from build123d import *

# Parameters (mm, degrees)
F0_W     = 10
F0_H     = 20
F1_DEPTH = 5
F2_R     = 1.5
F2_R_2   = 2.5
F3_DEPTH = 5
F4_R     = 1


with BuildPart() as f1:
    # F0 (on Top) → F1 (new body)
    with BuildSketch(Plane.XY):
        Rectangle(F0_W, F0_H)
    extrude(amount=F1_DEPTH)

    # F2 (on face) → F3 (join)
    with BuildSketch(Plane.XY.offset(5)):
        with Locations((0, 5.30432)):
            Circle(F2_R)
        with Locations((0, -5.19385)):
            Circle(F2_R_2)
    extrude(amount=F3_DEPTH)

    # F4
    f4_edges = [f1.edges().sort_by_distance(p)[0] for p in [
        (5, 0, 5),
        (0, -10, 5),
        (5, -10, 2.5),
        (5, 10, 2.5),
        (5, 0, 0),
        (-5, 0, 5),
        (0, 10, 5),
        (0, -10, 0),
        (0, 10, 0),
        (-5, 0, 0),
        (-5, -10, 2.5),
        (-5, 10, 2.5),
        (-2.5, -5.19385, 10),
        (-1.5, 5.30432, 10),
        (-1.5, 5.30432, 5),
        (-2.5, -5.19385, 5),
    ]]
    fillet(f4_edges, radius=F4_R)


solid = f1.part
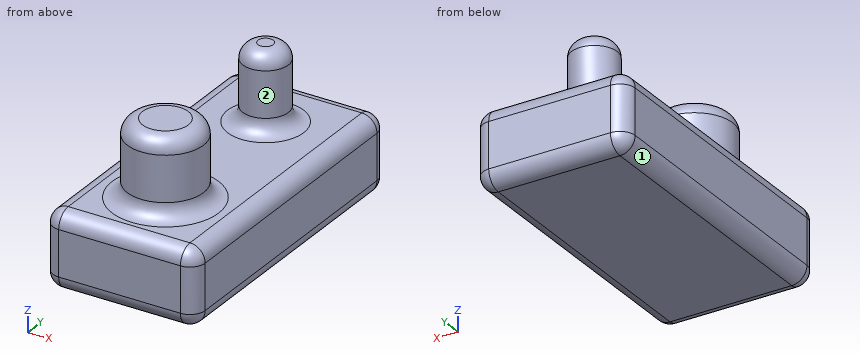
Geometry check sheet. Reference: the model listing, model coordinates, mm. Face numbers are marked on the shaded views. A direction names the side the tool comes from. Give positions to 0.01 mm unless a question says otherwise; leave off trailing zeros. Loops run counter-clockwise (first coordinate to the right, second up) from the corner with the lowest first, then second, coordinate; pieces in that order, holes last. Notation, with made-up numbers: M 10.5,-7.75 L 58.5,-7.75 A16 cw 58.5,17.25 Z; hole C 24,3.25 d11. An arc over 180 degrees is marked long. Write each question's results on one line, items separated by ' | '.
1) Gauge pin test, flat ends, axial feed: pin 1 (3 mm diameter, centred on x = -3, z = 6, fed in from +Y); pin 2 (1 mm diameter, centred on x = -2.5, z = 8, fed in from +Y). Record the tip position at first contact, or that the pin passes through.
Answers follow:
pin 1: y = 9.87 | pin 2: y = -3.69
2) Section check A-A, the plane y = 1. Record the boundary of the cut face in (x, z).
Answers follow:
outline: M -5,1 A1 ccw -4,0 L 4,0 A1 ccw 5,1 L 5,4 A1 ccw 4,5 L -4,5 A1 ccw -5,4 Z
3) Tool access check on the marked faces 1 and 2. Record the directions out of +Z, -Z, +X, -X, +Y, -Y that give a thin tool (end or side, any length) a straight path to the whole face; none if there is none.
Answers follow:
face 1: -Z, -X, +Y, -Y | face 2: +Z
4) Section check B-B, the plane z = 7. Record the boundary of the cut face in (x, y), plus the area to 3 significant figures.
Answers follow:
outline: C 0,-5.19 d5; C 0,5.3 d3 | area: 26.7 mm2
5) Thickness scan on line 1 (Z direction, x = -3.5, y = 1.75); line 2 (Z direction, x = 4.75, y = 6.75); line 3 (X direction, y = 6, z = 4.5). Record the ranges inside material, lowest first.
Answers follow:
line 1: 0 to 5 | line 2: 0.34 to 4.66 | line 3: -4.87 to 4.87
6) Section check C-C, the plane x = 4.5. Record the boundary of the cut face in (y, z), plus the area to 3 significant figures.
Answers follow:
outline: M -9.87,1 A0.87 ccw -9,0.13 L 9,0.13 A0.87 ccw 9.87,1 L 9.87,4 A0.87 ccw 9,4.87 L -9,4.87 A0.87 ccw -9.87,4 Z | area: 92.7 mm2
